Could you check a few things on this model? Use its own coordinates, in mm. A direction names the side the tool comes from. Give positions to 0.01 mm unless a question says otherwise; leave off trailing zeros. Write each loop counter-clockwise with the first axis right and the second up, starting at its lowest first coordinate (ties: lowest second). Pieces come first, ordered by that corner, then holes. Notation, with made-up numbers: (81.5, 15) -> (132.5, 15) arc R23 cw to (132.5, 51) -> close; hole circle Ø3 at (-23, 48.5). An arc over 180 degrees is marked (long way). Write item = value, one per line. Start each with the question number.
```python
from build123d import *

# Parameters (mm, degrees)
F0_R     = 9.525
F0_R_2   = 4.7625
F1_DEPTH = 3.175
F2_R     = 4.7625
F3_DEPTH = 6.35


# Not quite as in the source:
# - a feature names something its author has since deleted; it is built from what else it names


with BuildPart() as f1:
    # F0 (on Front) → F1 (new body)
    with BuildSketch(Plane.XZ):
        with Locations((-49.2760017514, 2.0293546841)):
            Circle(F0_R)
        with Locations((-49.2760017514, 2.0293546841)):
            Circle(F0_R_2, mode=Mode.SUBTRACT)
    extrude(amount=F1_DEPTH)

    # F2 (on face) → F3 (join)
    with BuildSketch(Plane.XZ.offset(3.175)):
        Polygon((-39.8072749816, 0.9955082934), (-43.6463011287, 9.7125894129), (-53.1150278984, 10.7464358035), (-58.7447285212, 3.0632010747), (-54.9057023742, -5.6538800448), (-45.4369756044, -6.6877264354), align=None)
        with Locations((-49.2760017514, 2.0293546841)):
            Circle(F2_R, mode=Mode.SUBTRACT)
    extrude(amount=F3_DEPTH)


solid = f1.part
```
(1) On a 3-axis mill with a long thin cutter (end or side, diameter ignored), from which of +Z, -Z, +X, -X, +Y, -Y can I reach the whole of each face in a straight line? I mean faces 1 (the flat face through (-41, -3.175, 6)), 2 (the flat face through (-55.89, -6.31, 6.96)), 3 (the flat face through (-42.66, -6.31, -2.9)), 4 (the flat face through (-57, -3.175, -2)). Say none if no direction works.
(2) Imagine slicing it at A-A (z = 0.25). Please give me the cut outline in (x, y) (3 decimals), then the cut area to 3 significant figures.
(3) I'm going to push flat-ended pins straight in: pin 1 (2 mm diameter, centred on x = -54, y = -2, fed in from -Z); pin 2 (1.5 mm diameter, centred on y = -7, z = 7.5, fed in from +X); pin 3 (4 mm diameter, centred on y = -8.5, z = 3, fed in from -X). Where does each tip first touch, or does it pass through?
(4) We'd pull the mould along Z, two halves only. Please class faces 5 (the cylindrical face through (-54.034, -4.696, 2.239)), 6 (the flat face through (-56.852, -6.306, -1.234)), 7 (the flat face through (-56.4, -3.175, 7.2)): released by +Z, released by -Z, zero draft, split by the parting line, or undercut.
(5) Imagine slicing it at B-B (x = -50). Please give me the cut outline in (y, z) (1 decimal), then the cut area to 3 significant figures.
(6) Imagine slicing it at C-C (y = -6.5). Please give me the cut outline in (x, z) (1 decimal), then the cut area to 3 significant figures.
(7) Imagine slicing it at D-D (x = -56). Please give me the cut outline in (y, z) (3 decimals).
(8) If I drill on line 1 along Z through (x, y) = (-51.75, -5.75); line 2 along X through (y, z) = (-1, 2.25); line 3 along Z through (x, y) = (-51.5, -7.25), over which ranges is the centre line in solid material (lowest first)? Write a range as from..to.
Answers below:
q1.face_1 = +Z, +X, -Y
q1.face_2 = +Z, -X, -Y
q1.face_3 = -Z, +X, -Y
q1.face_4 = -Z, -X, -Y
q2.outline = (-58.633, -3.175) -> (-57.506, -3.175) -> (-57.506, -9.525) -> (-53.694, -9.525) -> (-53.694, 0) -> (-58.633, 0) -> close; (-44.858, -9.525) -> (-40.354, -9.525) -> (-40.354, -3.175) -> (-39.919, -3.175) -> (-39.919, 0) -> (-44.858, 0) -> close
q2.area = 84.2 mm^2
q3.pin_1 = -6.74
q3.pin_2 = -42.34
q3.pin_3 = -58.74
q4.face_5 = undercut
q4.face_6 = released by -Z
q4.face_7 = zero draft
q5.outline = (-9.5, -6.2) -> (-3.2, -6.2) -> (-3.2, -7.5) -> (0, -7.5) -> (0, -2.7) -> (-9.5, -2.7) -> close; (-9.5, 6.7) -> (0, 6.7) -> (0, 11.5) -> (-3.2, 11.5) -> (-3.2, 10.4) -> (-9.5, 10.4) -> close
q5.area = 76.0 mm^2
q6.outline = (-58.7, 3.1) -> (-54.9, -5.7) -> (-45.4, -6.7) -> (-39.8, 1) -> (-43.6, 9.7) -> (-53.1, 10.7) -> close; hole circle Ø9.5 at (-49.3, 2)
q6.area = 164 mm^2
q7.outline = (-9.525, -3.169) -> (-3.175, -3.169) -> (-3.175, -4.717) -> (0, -4.717) -> (0, 8.776) -> (-3.175, 8.776) -> (-3.175, 6.809) -> (-9.525, 6.809) -> close
q8.line_1 = -6..-2.04, 6.1..10.6
q8.line_2 = -58.8..-54.03, -44.52..-39.75
q8.line_3 = -6.03..-2.18, 6.24..10.57
